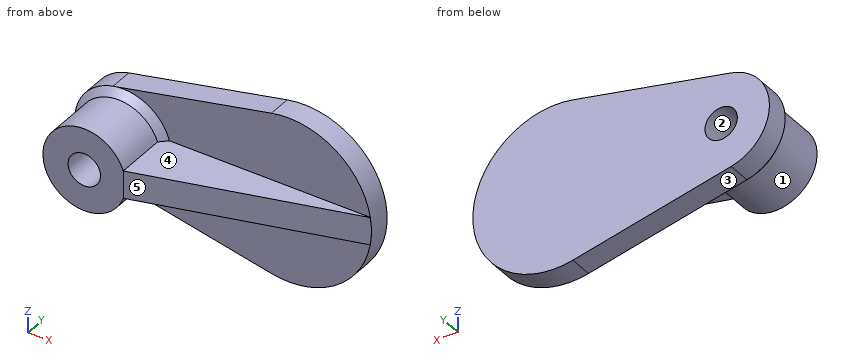
from build123d import *

# Parameters (mm, degrees)
SKETCH1_R               = 3
SKETCH1_R_2             = 1.175
BOSS_EXTRUDE1_DEPTH     = 5.9
BOSS_EXTRUDE2_START     = -1.7
SKETCH3_R               = 1.175
BOSS_EXTRUDE2_DEPTH     = 1.7
BOSS_EXTRUDE3_START     = 4.2
BOSS_EXTRUDE3_DEPTH     = 4.2
CUT_EXTRUDE1_DEPTH      = 20.869826371
CUT_EXTRUDE1_DEPTH_BACK = 20.869826371
CHAMFER2_SIZE           = 0.5


with BuildPart() as part:
    # Sketch1 → Boss-Extrude1 (new body)
    with BuildSketch(Plane(origin=(0, 0, 0), x_dir=(1, 0, 0), z_dir=(0, 1, 0))):
        with Locations(Location((0, 0, 0), (0, 0, 270))):
            Circle(SKETCH1_R)
        with Locations(Location((0, 0, 0), (0, 0, 270))):
            Circle(SKETCH1_R_2, mode=Mode.SUBTRACT)
    extrude(amount=BOSS_EXTRUDE1_DEPTH)

    # Sketch3 → Boss-Extrude2 (add)
    with BuildSketch(Plane(origin=(0, 5.9, 0), x_dir=(1, 0, 0), z_dir=(0, 1, 0)).offset(BOSS_EXTRUDE2_START)):
        with BuildLine():
            Line((-0.729166667, 3.42320259), (10.75, 5.868347297))
            ThreePointArc((10.75, 5.868347297), (18, 0), (10.75, -5.868347297))
            Line((10.75, -5.868347297), (-0.729166667, -3.42320259))
            ThreePointArc((-0.729166667, -3.42320259), (-3.5, 0), (-0.729166667, 3.42320259))
        make_face()
        with Locations(Location((0, 0, 0), (0, 0, 270))):
            Circle(SKETCH3_R, mode=Mode.SUBTRACT)
    extrude(amount=BOSS_EXTRUDE2_DEPTH)

    # Sketch4 → Boss-Extrude3 (add)
    with BuildSketch(Plane.XZ.offset(-4.2).offset(BOSS_EXTRUDE3_START)):
        with BuildLine():
            Line((2.828427125, 1), (17.916079783, 1))
            ThreePointArc((17.916079783, 1), (18, 0), (17.916079783, -1))
            Line((17.916079783, -1), (2.828427125, -1))
            ThreePointArc((2.828427125, -1), (3, 0), (2.828427125, 1))
        make_face()
    extrude(amount=-BOSS_EXTRUDE3_DEPTH)

    # Sketch5 → Cut-Extrude1 (cut, two sides: drawn at the far end of the back side and taken through both)
    with BuildSketch(Plane.XY.offset(-CUT_EXTRUDE1_DEPTH_BACK)):
        Polygon((2.828427125, 0), (18, 4.2), (18, 0), align=None)
    extrude(amount=CUT_EXTRUDE1_DEPTH + CUT_EXTRUDE1_DEPTH_BACK, mode=Mode.SUBTRACT)

    # Chamfer2
    chamfer2_edges = [part.edges().sort_by_distance(p)[0] for p in [
        (-3, 4.2, 0),
    ]]
    chamfer(chamfer2_edges, length=CHAMFER2_SIZE - 0.0001)  # a hair under: the kernel refuses the full size


solid = part.part
Here's how the part is built. I have some questions about the finished solid (model axes, mm). Face numbers are marked on the shaded views. A direction names the side the tool comes from. Give positions to 0.01 mm unless a question says otherwise; leave off trailing zeros. Order: outer loops, then holes, each group sorted by start corner. A loop starts at its lowest first (then second) coordinate and runs counter-clockwise, first axis right, second up. Notation, with made-up numbers: M 40.5,85.5 L 75.5,85.5 A30 ccw 75.5,120.5 Z; hole C 31,20 d3. An arc over 180 degrees is marked long. Answer as a JSON object with one key per item and string values. Group by question number.
1) I'm going to push flat-ended pins straight in: pin 1 Ø1 at (y, z) = (1, -4.5) entering from -X; pin 2 Ø1.5 at (y, z) = (4.5, 1) entering from +X; pin 3 Ø1.5 at (x, y) = (7, 1) entering from -Z; pin 4 Ø2.5 at (x, z) = (0, 0) entering from -Y. Where does each tip first touch, or does it pass through?
2) Suppose I cut it at C-C, the plane x = 6. Write out the boundary of the cut face in (y, z).
3) On a 3-axis mill with a long thin cutter (end or side, diameter ignored), from which of +Z, -Z, +X, -X, +Y, -Y can I reach the whole of each face in a straight line? I mean the marked faces 4 and 5. Say none if no direction works.
4) Suppose I cut it at B-B, the plane y = 1.1. Write out the boundary of the cut face in (x, z) (3 decimals).
5) Please list where these lines run through material, in increasing order: L1, parallel to Y at x = 8.25, z = 1.5; L2, parallel to Z at x = 7, y = 1.6; L3, parallel to Z at x = 0.75, y = 2.1. Write a range as [from, to].
6) Suppose I cut it at A-A, the plane x = 0. Write out the boundary of the cut face in (y, z) (3 decimals), plus the area to 3 significant figures.
7) Suppose I cut it at D-D, the plane z = -4. Write out the boundary of the cut face in (x, y), plus the area to 3 significant figures.
8) We'd pull the mould along Z, two halves only. Please class the marked faces 1, 2 and 3: pulls with the +Z half, pulls with the -Z half, needs draft (parallel to the pull), parting line crosses it, or undercut.
Results found:
{
 "1": {"pin 1": "through", "pin 2": "x = 17.99", "pin 3": "z = -1", "pin 4": "y = 0"},
 "2": {"outline": "M 0.88,-1 L 4.2,-1 L 4.2,-4.86 L 5.9,-4.86 L 5.9,4.86 L 4.2,4.86 L 4.2,1 L 0.88,1 Z"},
 "3": {"face 4": "+Z, +X, -Y", "face 5": "+Z, -Z, +X, -Y"},
 "4": {"outline": "M 2.828,-1 L 6.802,-1 L 6.802,1 L 2.828,1 A3 ccw long Z; hole C 0,0 d2.35"},
 "5": {"L1": "[4.2, 5.9]", "L2": "[-1, 1]", "L3": "[-2.9, -0.9], [0.9, 2.9]"},
 "6": {"outline": "M 0,-3 L 3.7,-3 L 4.2,-3.5 L 4.2,-3.579 L 5.9,-3.579 L 5.9,-1.175 L 0,-1.175 Z; M 0,1.175 L 5.9,1.175 L 5.9,3.579 L 4.2,3.579 L 4.2,3.5 L 3.7,3 L 0,3 Z", "area": "23.8 mm²"},
 "7": {"outline": "M 1.98,4.2 L 16.47,4.2 L 16.47,5.9 L 1.98,5.9 Z", "area": "24.6 mm²"},
 "8": {"face 1": "parting line crosses it", "face 2": "undercut", "face 3": "pulls with the -Z half"}
}
